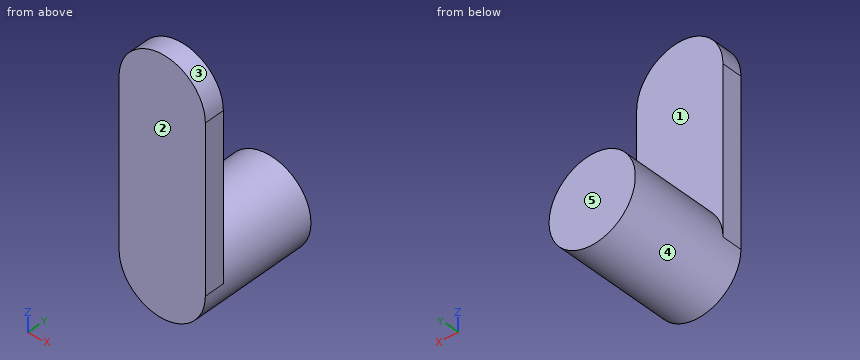
```python
from build123d import *

# Parameters (mm, degrees)
F1_DEPTH = 108.966
F2_DEPTH = 18.542


with BuildPart() as f1:
    # F0 (on Front) → F1 (new body)
    with BuildSketch(Plane.XZ):
        with BuildLine():
            ThreePointArc((-39.341677, -77.595275), (0, -116.936952), (39.341677, -77.595275))
            Line((39.341677, -77.595275), (-39.341677, -77.595275))
        make_face()
        with BuildLine():
            Line((-39.341677, -77.595275), (39.341677, -77.595275))
            ThreePointArc((39.341677, -77.595275), (0, -38.253598), (-39.341677, -77.595275))
        make_face()
    extrude(amount=-F1_DEPTH)

    # F0 (on Front) → F2 (join)
    with BuildSketch(Plane.XZ):
        with BuildLine():
            Line((39.341677, -77.595275), (39.341677, 72.270408))
            ThreePointArc((39.341677, 72.270408), (0, 32.928731), (-39.341677, 72.270408))
            Line((-39.341677, 72.270408), (-39.341677, -77.595275))
            ThreePointArc((-39.341677, -77.595275), (0, -38.253598), (39.341677, -77.595275))
        make_face()
        with BuildLine():
            ThreePointArc((-39.341677, 72.270408), (0, 32.928731), (39.341677, 72.270408))
            Line((39.341677, 72.270408), (-39.341677, 72.270408))
        make_face()
        with BuildLine():
            Line((-39.341677, 72.270408), (39.341677, 72.270408))
            ThreePointArc((39.341677, 72.270408), (0, 111.612085), (-39.341677, 72.270408))
        make_face()
    extrude(amount=-F2_DEPTH)


solid = f1.part
```
Could you check a few things on this model? Use its own coordinates, in mm. Face numbers are marked on the shaded views. A direction names the side the tool comes from. Give positions to 0.01 mm unless a question says otherwise; leave off trailing zeros. Loops run counter-clockwise (first coordinate to the right, second up) from the corner with the lowest first, then second, coordinate; pieces in that order, holes last. Notation, with made-up numbers: (2.5, 10.5) -> (12.5, 10.5) arc R31 ccw to (12.5, 40.5) -> close; hole circle Ø2 at (-24.5, 7.25). An arc over 180 degrees is marked (long way). Put each result on its own line as item: value.
(1) Imagine slicing it at D-D on x = 21. Write out the boundary of the cut face in (y, z).
Computed:
outline: (0, -110.86) -> (108.97, -110.86) -> (108.97, -44.33) -> (18.54, -44.33) -> (18.54, 105.54) -> (0, 105.54) -> close
(2) Imagine slicing it at C-C on z = 14. Write out the boundary of the cut face in (x, y).
Computed:
outline: (-39.34, 0) -> (39.34, 0) -> (39.34, 18.54) -> (-39.34, 18.54) -> close
(3) Imagine slicing it at B-B on x = 0. Write out the boundary of the cut face in (y, z).
Computed:
outline: (0, -116.94) -> (108.97, -116.94) -> (108.97, -38.25) -> (18.54, -38.25) -> (18.54, 111.61) -> (0, 111.61) -> close
(4) Imagine slicing it at A-A on y = 41.5. Write out the boundary of the cut face in (x, z), plus the area to 3 significant figures.
Computed:
outline: circle Ø78.68 at (0, -77.6)
area: 4,860 mm^2
(5) Please list where these lines run through material, in increasing order: probe 1 along Y at (x, z) = (-14.5, 93); probe 2 along Z at (x, y) = (-1, 88); probe 3 along Z at (x, y) = (23.5, 63.5). Write a range as [from, to].
Computed:
probe 1: [0, 18.54]
probe 2: [-116.92, -38.27]
probe 3: [-109.15, -46.04]
(6) Thinking about a two-plate mould opening in Y: for the marked faces 1, 2 and 3, which applies, pulls with the +Y half, pulls with the -Y half, needs draft (parallel to the pull), parting line crosses it, or undercut?
Computed:
face 1: pulls with the +Y half
face 2: pulls with the -Y half
face 3: needs draft
(7) I'm going to push flat-ended pins straight in: pin 1 Ø23.5 at (x, z) = (-4, -21) entering from +Y; pin 2 Ø8 at (y, z) = (17.5, 81.5) entering from -X; pin 3 Ø8 at (x, y) = (29, 42.5) entering from +Z. Where does each tip first touch, or does it pass through?
Computed:
pin 1: y = 18.54
pin 2: x = -38.99
pin 3: z = -47.22
(8) For the marked faces 4 and 5, which set-ups out of +Z, -Z, +X, -X, +Y, -Y let a thin tool reach every point of the face, with its end or its side?
Computed:
face 4: +Y
face 5: +Z, -Z, +X, -X, +Y
